from build123d import *

# Parameters (mm, degrees)
F0_R     = 1.5
F1_DEPTH = 1.5


with BuildPart() as f1:
    # F0 (on Top) → F1 (new body)
    with BuildSketch(Plane.XY):
        with BuildLine():
            ThreePointArc((-25.3176430492, 29.4941114099), (-25.0810531663, 28.9761945322), (-25, 28.4125962273))
            Line((-25, 28.4125962273), (-25, -28.4125962273))
            ThreePointArc((-25, -28.4125962273), (-25.0810531663, -28.9761945322), (-25.3176430492, -29.4941114099))
            Line((-25.3176430492, -29.4941114099), (-33.4704606701, -42.1762721535))
            ThreePointArc((-33.4704606701, -42.1762721535), (-33.774657608, -43.026262721), (-33.6740843865, -43.9234275716))
            Line((-33.6740843865, -43.9234275716), (-25.0442624935, -68.3745896019))
            ThreePointArc((-25.0442624935, -68.3745896019), (-25.0086166049, -68.5018102431), (-24.9900535171, -68.6326197714))
            Line((-24.9900535171, -68.6326197714), (-23.6174713638, -86.9337151489))
            ThreePointArc((-23.6174713638, -86.9337151489), (-23.0992020506, -88.1335952445), (-21.9505091584, -88.7571495439))
            Line((-21.9505091584, -88.7571495439), (-0.3274364143, -92.3456594887))
            ThreePointArc((-0.3274364143, -92.3456594887), (0, -92.3726451972), (0.3274364143, -92.3456594887))
            Line((0.3274364143, -92.3456594887), (21.9505091584, -88.7571495439))
            ThreePointArc((21.9505091584, -88.7571495439), (23.0992020506, -88.1335952445), (23.6174713638, -86.9337151489))
            Line((23.6174713638, -86.9337151489), (24.9900535171, -68.6326197714))
            ThreePointArc((24.9900535171, -68.6326197714), (25.0086166049, -68.5018102431), (25.0442624935, -68.3745896019))
            Line((25.0442624935, -68.3745896019), (33.6740843865, -43.9234275716))
            ThreePointArc((33.6740843865, -43.9234275716), (33.774657608, -43.026262721), (33.4704606701, -42.1762721535))
            Line((33.4704606701, -42.1762721535), (25.3176430492, -29.4941114099))
            ThreePointArc((25.3176430492, -29.4941114099), (25.0810531663, -28.9761945322), (25, -28.4125962273))
            Line((25, -28.4125962273), (25, 28.4125962273))
            ThreePointArc((25, 28.4125962273), (25.0810531663, 28.9761945322), (25.3176430492, 29.4941114099))
            Line((25.3176430492, 29.4941114099), (33.4704606701, 42.1762721535))
            ThreePointArc((33.4704606701, 42.1762721535), (33.774657608, 43.026262721), (33.6740843865, 43.9234275716))
            Line((33.6740843865, 43.9234275716), (25.0442624935, 68.3745896019))
            ThreePointArc((25.0442624935, 68.3745896019), (25.0086166049, 68.5018102431), (24.9900535171, 68.6326197714))
            Line((24.9900535171, 68.6326197714), (23.6174713638, 86.9337151489))
            ThreePointArc((23.6174713638, 86.9337151489), (23.0992020506, 88.1335952445), (21.9505091584, 88.7571495439))
            Line((21.9505091584, 88.7571495439), (0.3274364143, 92.3456594887))
            ThreePointArc((0.3274364143, 92.3456594887), (0, 92.3726451972), (-0.3274364143, 92.3456594887))
            Line((-0.3274364143, 92.3456594887), (-21.9505091584, 88.7571495439))
            ThreePointArc((-21.9505091584, 88.7571495439), (-23.0992020506, 88.1335952445), (-23.6174713638, 86.9337151489))
            Line((-23.6174713638, 86.9337151489), (-24.9900535171, 68.6326197714))
            ThreePointArc((-24.9900535171, 68.6326197714), (-25.0086166049, 68.5018102431), (-25.0442624935, 68.3745896019))
            Line((-25.0442624935, 68.3745896019), (-33.6740843865, 43.9234275716))
            ThreePointArc((-33.6740843865, 43.9234275716), (-33.774657608, 43.026262721), (-33.4704606701, 42.1762721535))
            Line((-33.4704606701, 42.1762721535), (-25.3176430492, 29.4941114099))
        make_face()
        with Locations((-24.2299033358, -56.7940851803)):
            Circle(F0_R, mode=Mode.SUBTRACT)
        with Locations((-15.875, -81.7)):
            Circle(F0_R, mode=Mode.SUBTRACT)
        with Locations((-14.8, -53.465884003)):
            Circle(F0_R, mode=Mode.SUBTRACT)
        with Locations((-28.2237447487, -45.4782011774)):
            Circle(F0_R, mode=Mode.SUBTRACT)
        with Locations((-18.7938414128, -42.15)):
            Circle(F0_R, mode=Mode.SUBTRACT)
        with Locations((-17.15, -30.1)):
            Circle(F0_R, mode=Mode.SUBTRACT)
        with BuildLine():
            Line((-14.1421356237, -16.2634559673), (-16.8291413922, -18.9504617358))
            ThreePointArc((-16.8291413922, -18.9504617358), (-18.9504617358, -18.9504617358), (-18.9504617358, -16.8291413922))
            Line((-18.9504617358, -16.8291413922), (-16.2634559673, -14.1421356237))
            ThreePointArc((-16.2634559673, -14.1421356237), (-14.1421356237, -14.1421356237), (-14.1421356237, -16.2634559673))
        make_face(mode=Mode.SUBTRACT)
        with Locations((15.875, -81.7)):
            Circle(F0_R, mode=Mode.SUBTRACT)
        with BuildLine():
            Line((-3.9, -57), (3.9, -57))
            ThreePointArc((3.9, -57), (4.6071067812, -57.2928932188), (4.9, -58))
            Line((4.9, -58), (4.9, -70.7))
            ThreePointArc((4.9, -70.7), (4.6071067812, -71.4071067812), (3.9, -71.7))
            Line((3.9, -71.7), (-3.9, -71.7))
            ThreePointArc((-3.9, -71.7), (-4.6071067812, -71.4071067812), (-4.9, -70.7))
            Line((-4.9, -70.7), (-4.9, -58))
            ThreePointArc((-4.9, -58), (-4.6071067812, -57.2928932188), (-3.9, -57))
        make_face(mode=Mode.SUBTRACT)
        with Locations((14.8, -53.465884003)):
            Circle(F0_R, mode=Mode.SUBTRACT)
        with Locations((24.2299033358, -56.7940851803)):
            Circle(F0_R, mode=Mode.SUBTRACT)
        with BuildLine():
            ThreePointArc((3.85, -20.2), (4.5571067812, -20.4928932188), (4.85, -21.2))
            Line((4.85, -21.2), (4.85, -37.1))
            ThreePointArc((4.85, -37.1), (4.5571067812, -37.8071067812), (3.85, -38.1))
            Line((3.85, -38.1), (-3.85, -38.1))
            ThreePointArc((-3.85, -38.1), (-4.5571067812, -37.8071067812), (-4.85, -37.1))
            Line((-4.85, -37.1), (-4.85, -21.2))
            ThreePointArc((-4.85, -21.2), (-4.5571067812, -20.4928932188), (-3.85, -20.2))
            Line((-3.85, -20.2), (3.85, -20.2))
        make_face(mode=Mode.SUBTRACT)
        with BuildLine():
            Line((16.2634559673, -14.1421356237), (18.9504617358, -16.8291413922))
            ThreePointArc((18.9504617358, -16.8291413922), (18.9504617358, -18.9504617358), (16.8291413922, -18.9504617358))
            Line((16.8291413922, -18.9504617358), (14.1421356237, -16.2634559673))
            ThreePointArc((14.1421356237, -16.2634559673), (14.1421356237, -14.1421356237), (16.2634559673, -14.1421356237))
        make_face(mode=Mode.SUBTRACT)
        with Locations((18.7938414128, -42.15)):
            Circle(F0_R, mode=Mode.SUBTRACT)
        with Locations((17.15, -30.1)):
            Circle(F0_R, mode=Mode.SUBTRACT)
        with Locations((28.2237447487, -45.4782011774)):
            Circle(F0_R, mode=Mode.SUBTRACT)
        with Locations((-28.2237447487, 45.4782011774)):
            Circle(F0_R, mode=Mode.SUBTRACT)
        with Locations((-17.15, 30.1)):
            Circle(F0_R, mode=Mode.SUBTRACT)
        with Locations((-18.7938414128, 42.15)):
            Circle(F0_R, mode=Mode.SUBTRACT)
        with BuildLine():
            Line((-16.2634559673, 14.1421356237), (-18.9504617358, 16.8291413922))
            ThreePointArc((-18.9504617358, 16.8291413922), (-18.9504617358, 18.9504617358), (-16.8291413922, 18.9504617358))
            Line((-16.8291413922, 18.9504617358), (-14.1421356237, 16.2634559673))
            ThreePointArc((-14.1421356237, 16.2634559673), (-14.1421356237, 14.1421356237), (-16.2634559673, 14.1421356237))
        make_face(mode=Mode.SUBTRACT)
        with Locations((-24.2299033358, 56.7940851803)):
            Circle(F0_R, mode=Mode.SUBTRACT)
        with Locations((-14.8, 53.465884003)):
            Circle(F0_R, mode=Mode.SUBTRACT)
        with Locations((-15.875, 81.7)):
            Circle(F0_R, mode=Mode.SUBTRACT)
        with BuildLine():
            ThreePointArc((-14.8, 7.8), (-14.5071067812, 8.5071067812), (-13.8, 8.8))
            Line((-13.8, 8.8), (13.8, 8.8))
            ThreePointArc((13.8, 8.8), (14.5071067812, 8.5071067812), (14.8, 7.8))
            Line((14.8, 7.8), (14.8, -7.8))
            ThreePointArc((14.8, -7.8), (14.5071067812, -8.5071067812), (13.8, -8.8))
            Line((13.8, -8.8), (-13.8, -8.8))
            ThreePointArc((-13.8, -8.8), (-14.5071067812, -8.5071067812), (-14.8, -7.8))
            Line((-14.8, -7.8), (-14.8, 7.8))
        make_face(mode=Mode.SUBTRACT)
        with BuildLine():
            ThreePointArc((16.8291413922, 18.9504617358), (18.9504617358, 18.9504617358), (18.9504617358, 16.8291413922))
            Line((18.9504617358, 16.8291413922), (16.2634559673, 14.1421356237))
            ThreePointArc((16.2634559673, 14.1421356237), (14.1421356237, 14.1421356237), (14.1421356237, 16.2634559673))
            Line((14.1421356237, 16.2634559673), (16.8291413922, 18.9504617358))
        make_face(mode=Mode.SUBTRACT)
        with BuildLine():
            Line((3.85, 19.4), (-3.85, 19.4))
            ThreePointArc((-3.85, 19.4), (-4.5571067812, 19.6928932188), (-4.85, 20.4))
            Line((-4.85, 20.4), (-4.85, 36.3))
            ThreePointArc((-4.85, 36.3), (-4.5571067812, 37.0071067812), (-3.85, 37.3))
            Line((-3.85, 37.3), (3.85, 37.3))
            ThreePointArc((3.85, 37.3), (4.5571067812, 37.0071067812), (4.85, 36.3))
            Line((4.85, 36.3), (4.85, 20.4))
            ThreePointArc((4.85, 20.4), (4.5571067812, 19.6928932188), (3.85, 19.4))
        make_face(mode=Mode.SUBTRACT)
        with Locations((17.15, 30.1)):
            Circle(F0_R, mode=Mode.SUBTRACT)
        with Locations((18.7938414128, 42.15)):
            Circle(F0_R, mode=Mode.SUBTRACT)
        with Locations((28.2237447487, 45.4782011774)):
            Circle(F0_R, mode=Mode.SUBTRACT)
        with BuildLine():
            Line((3.9, 56.2), (-3.9, 56.2))
            ThreePointArc((-3.9, 56.2), (-4.6071067812, 56.4928932188), (-4.9, 57.2))
            Line((-4.9, 57.2), (-4.9, 69.9))
            ThreePointArc((-4.9, 69.9), (-4.6071067812, 70.6071067812), (-3.9, 70.9))
            Line((-3.9, 70.9), (3.9, 70.9))
            ThreePointArc((3.9, 70.9), (4.6071067812, 70.6071067812), (4.9, 69.9))
            Line((4.9, 69.9), (4.9, 57.2))
            ThreePointArc((4.9, 57.2), (4.6071067812, 56.4928932188), (3.9, 56.2))
        make_face(mode=Mode.SUBTRACT)
        with Locations((14.8, 53.465884003)):
            Circle(F0_R, mode=Mode.SUBTRACT)
        with Locations((15.875, 81.7)):
            Circle(F0_R, mode=Mode.SUBTRACT)
        with Locations((24.2299033358, 56.7940851803)):
            Circle(F0_R, mode=Mode.SUBTRACT)
    extrude(amount=F1_DEPTH)


solid = f1.part
Work out the finished part from the listing and answer in its coordinate system (mm). A direction names the side the tool comes from. Round coordinates to 2 decimals unless told otherwise and drop trailing zeros. Write each loop counter-clockwise with the first axis right and the second up, starting at its lowest first coordinate (ties: lowest second). Pieces come first, ordered by that corner, then holes. Notation, with made-up numbers: (34.5, 21.25) - (69.5, 21.25) arc R24 ccw to (69.5, 37.25) - close; hole circle Ø3 at (52, 32.5). An arc over 180 degrees is marked (long way). Answer in a Markdown table with one row per item. Add a question column.
1. A cutting plane is placed at D-D, the plane y = 39. Determine the outline of the cut face in (x, z), and give its area (3 significant figures).
2. A cutting plane is placed at A-A, the plane x = -6.5. Determine the outline of the cut face in (y, z).
3. For faces 4 (the cylindrical face through (17.84, 28.77, 0.74)), 5 (the flat face through (-29.34, -35.75, 0.74)), determine the directions among +Z, -Z, +X, -X, +Y, -Y from which every point of the face is accessible in a straight line to the end or side of a thin tool.
4. Given pin 1 (1.8 mm diameter, centred on x = -14.8, y = 53.47, fed in from -Z); pin 2 (0.8 mm diameter, centred on y = 2.5, z = 1, fed in from -X); pin 3 (0.8 mm diameter, centred on x = 3, z = 1, fed in from +Y), each flat-ended and moving along its own axis, determine where each tip first touches the part or whether it passes through.
5. A cutting plane is placed at C-C, the plane z = 0.55. Count the separate pieces of the cut face and the enclosed holes in it, and give its area (3 significant figures).
6. A cutting plane is placed at B-B, the plane x = 10. Determine the outline of the cut face in (y, z).
7. Find the intervals of material crossed by line 1 along X through (y, z) = (-28, 1.15); line 2 along X through (y, z) = (-42, 0.7); line 3 along X through (y, z) = (-3.5, 0.95), in increasing order. Write a range as from..to.
8. The mould has two halves that part along Y. Classify faces 1 (the flat face through (-29.3, 56.32, 0.74)), 2 (the flat face through (-15, 1, 0)), 3 (the cylindrical face through (17.84, -31.43, 0.74)): +Y half, -Y half, draft (parallel to the pull), parting line (faces both ways), or undercut.
Worked out:
| question | item | result |
|---|---|---|
| 1 | outline | (-31.43, 0) - (31.43, 0) - (31.43, 1.5) - (-31.43, 1.5) - close |
| 1 | area | 94.3 mm^2 |
| 2 | outline | (-91.32, 0) - (-8.8, 0) - (-8.8, 1.5) - (-91.32, 1.5) - close; (8.8, 0) - (91.32, 0) - (91.32, 1.5) - (8.8, 1.5) - close |
| 3 | face 4 | +Z, -Z |
| 3 | face 5 | +Z, -Z, -X |
| 4 | pin 1 | through |
| 4 | pin 2 | x = -25 |
| 4 | pin 3 | y = 91.97 |
| 5 | separate pieces | 1 |
| 5 | enclosed holes | 33 |
| 5 | area | 8,290 mm^2 |
| 6 | outline | (-90.74, 0) - (-8.8, 0) - (-8.8, 1.5) - (-90.74, 1.5) - close; (8.8, 0) - (90.74, 0) - (90.74, 1.5) - (8.8, 1.5) - close |
| 7 | line 1 | -25..-4.85, 4.85..25 |
| 7 | line 2 | -33.36..-20.29, -17.3..17.3, 20.29..33.36 |
| 7 | line 3 | -25..-14.8, 14.8..25 |
| 8 | face 1 | +Y half |
| 8 | face 2 | draft |
| 8 | face 3 | undercut |
